Autodesk Inventor part; units mm, degrees
ref_plane "YZ Plane" through (0, 0, 0) normal (1, 0, 0) x (0, 1, 0)
ref_plane "XZ Plane" through (0, 0, 0) normal (0, 1, 0) x (-1, 0, 0)
ref_plane "XY Plane" through (0, 0, 0) normal (0, 0, 1) x (1, 0, 0)
sketch "Sketch1" plane through (0, 0, 0) normal (0, 0, 1) x (1, 0, 0)
  line L0 (25, 0) -> (30, 0)
  line L1 (30, 0) -> (30, 100)
  line L2 (30, 100) -> (55, 100)
  line L3 (55, 100) -> (55, 95)
  line L4 (55, 95) -> (60, 95)
  line L5 (60, 95) -> (60, 105)
  line L6 (60, 105) -> (30, 105)
  line L7 (30, 105) -> (30, 395)
  line L8 (30, 395) -> (0, 395)
  line L9 (0, 250) -> (0, 395)
  line L10 (25, 0) -> (25, 250)
  line L11 (25, 250) -> (0, 250)
  line L12 (0, 0) -> (0, 395)
  dimension "d0" = 25
  dimension "d1" = 5
  dimension "d2" = 100
  dimension "d3" = 25
  dimension "d4" = 5
  dimension "d5" = 5
  dimension "d6" = 10
  dimension "d7" = 290
  dimension "d8" = 250
revolve "Revolution1" add sketch "Sketch1" angle 360 mid plane about axis through (0, 0, 0) along (0, 1, 0)
fillet "Fillet1" radius 5 3 edges at (30, 105, 0) (60, 105, 0) (30, 100, 0)
sketch "Sketch2" plane through (0, 395, 0) normal (0, 1, 0) x (1, 0, 0)
  line L0 (15, 0) -> (-15, 0)
  circle A0 centre (0, 0) radius 25
  circle A1 centre (0, 0) radius 30
  line L1 (-15, -25.9808) -> (-15, 25.9808)
  line L2 (15, 0) -> (15, -25.9808)
  line L3 (15, -25.9808) -> (15, 25.9808)
  arc A2 (15, 25.9808) -> (-15, 25.9808) centre (0, 0) ccw
  arc A3 (-15, -25.9808) -> (15, -25.9808) centre (0, 0) ccw
  dimension "d11" = 15
  dimension "d12" = 30
extrude "Extrusion1" add sketch "Sketch2" along normal blind 35 contours L2 A0 L1 L0 | L0 L1 A0 L3 | L2 A1 L1 A0 | A0 L1 A1 L3
fillet "Fillet2" radius 2 4 edges at (-15, 430, 0) (15, 430, 12.9904) (0, 430, -30) (0, 430, 30)
fillet "Fillet3" radius 5 2 edges at (-15, 395, 0) (15, 395, 12.9904)
sketch "Sketch3" plane through (-15, 428, -25.9808) normal (-1, 0, 0) x (0, 0, 1)
  line L0 (0, -28) -> (0, 0)
  line L1 (0, 0) -> (51.9615, 0)
  line L2 (0, -28) -> (51.9615, -28)
  circle A0 centre (25.9808, -14) radius 10
  point P0 (25.9808, -428)
  dimension "d17" = 20
hole "Hole1" at (-15, 414, 0) direction (1, 0, 0) diameter 20 end through all
fillet "Fillet4" radius 2 1 edges at (30, 0, 0)
properties part number "shield" material "Steel, High Strength, Low Alloy"
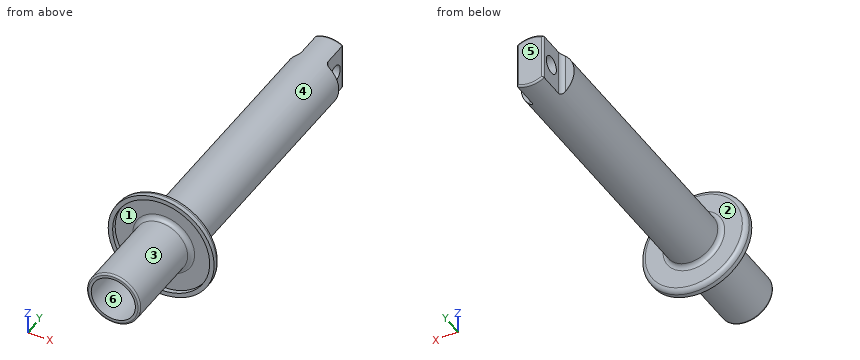
Read the model definition and answer for the solid it produces. Units are mm, in the model's axes. Face numbers are marked on the shaded views. A direction names the side the tool comes from. Give positions to 0.01 mm unless a question says otherwise; leave off trailing zeros. Loops run counter-clockwise (first coordinate to the right, second up) from the corner with the lowest first, then second, coordinate; pieces in that order, holes last. Notation, with made-up numbers: (16, -9) - (29, -9) arc R15 cw to (29, 16) - close; hole circle Ø5 at (22.25, 89.25). An arc over 180 degrees is marked (long way). Answer as CSV lines item,"result". Start each with the question number.
1) Determine the mould class of the marked faces 1, 2 and 3 for opening direction Z: released by +Z, released by -Z, zero draft, split by the parting line, or undercut.
2) Each of these flat-tipped pins is pushed along its axis until it touches: pin 1 Ø4 at (x, z) = (39.5, -38.5) entering from +Y; pin 2 Ø1 at (x, z) = (11, 43.5) entering from -Y; pin 3 Ø1 at (x, y) = (-15.5, 211) entering from +Z. Where does it stop, or does it pass through?
3) Find section C-C (y = 414). Write down the section's boundary in (x, z), then the cut area to 3 significant figures.
4) Straight lines are drawn through the part: L1, parallel to Z at x = -1, y = 414; L2, parallel to Z at x = 0, y = 98.55; L3, parallel to Y at x = 8, z = 0. For each, find the intervals that lie inside material, in ascending order. Write a range as from..to.
5) Which of the six approach directions +Z, -Z, +X, -X, +Y, -Y give full straight-line access (tool end or side, diameter ignored) to the marked faces 4, 5 and 6?
6) Find section B-B (y = 165). Write down the section's boundary in (x, z), then the cut area to 3 significant figures.
7) Find section D-D (y = 328). Write down the section's boundary in (x, z).
Findings below:
1,face 1,"undercut"
1,face 2,"zero draft"
1,face 3,"split by the parting line"
2,pin 1,"y = 105"
2,pin 2,"y = 100"
2,pin 3,"z = 25.98"
3,outline,"(-15, -25.98) arc R30 ccw to (15, -25.98) - (15, -10) - (-15, -10) - close; (-15, 10) - (15, 10) - (15, 25.98) arc R30 ccw to (-15, 25.98) - close"
3,area,"1,120 mm^2"
4,L1,"-29.98..-10, 10..29.98"
4,L2,"-60..-55, -31.48..-25, 25..31.48, 55..60"
4,L3,"250..404, 424..430"
5,face 4,"+Y"
5,face 5,"+Z, -Z, +X, -X, +Y"
5,face 6,"-Y"
6,outline,"circle Ø60 at (0, 0); hole circle Ø50 at (0, 0)"
6,area,"864 mm^2"
7,outline,"circle Ø60 at (0, 0)"
